from build123d import *

# Parameters (mm, degrees)
F1_DEPTH  = 22.5
F3_W      = 26.150945574
F3_H      = 2.773584798
F4_DEPTH  = 18
F7_R      = 5
F6_W      = 35.4622639716
F6_H      = 18.6226405203
F8_DEPTH  = 1.5
F10_R     = 2.7697383404
F11_DEPTH = 1.5
F14_R     = 2.5
F15_DEPTH = 1.3
F17_R     = 2.6497529256
F18_DEPTH = 1.5


# Not quite as in the source:
# - a pattern or mirror of a feature is missing from the dataset's text; its kind, count and spacing are read off the source's solid


with BuildPart() as f1:
    # F0 (on Front) → F1 (new body, symmetric)
    with BuildSketch(Plane.XZ):
        Polygon((9.8066031933, -27.5377351791), (14.9575471878, -27.5377351791), (14.9575471878, 27.5377351791), (-14.9575471878, 27.5377351791), (-14.9575471878, -27.5377351791), (2.2783020977, -27.5377351791), (2.2783020977, -14.8584917188), (9.8066031933, -14.8584917188), align=None)
    extrude(amount=F1_DEPTH, both=True)

    # F3 (on offset) → F4 (cut)
    with BuildSketch(Plane.XY.offset(27.5377351791)):
        with Locations((0, 15.5518874526)):
            Rectangle(F3_W, F3_H)
        with Locations((0, 5.5518874526)):
            Rectangle(F3_W, F3_H)
        with Locations((0, -4.4481125474)):
            Rectangle(F3_W, F3_H)
        with Locations((0, -14.4481125474)):
            Rectangle(F3_W, F3_H)
    extrude(amount=-F4_DEPTH, mode=Mode.SUBTRACT)

    # F7
    f7_edges = [f1.edges().sort_by_distance(p)[0] for p in [
        (0, -22.5, 27.537735),
        (0, 22.5, 27.537735),
    ]]
    fillet(f7_edges, radius=F7_R)

    # F6 (on offset) → F8 (cut)
    with BuildSketch(Plane(origin=(-14.9575471878, 0, 0), x_dir=(0, -1, 0), z_dir=(-1, 0, 0))):
        with Locations((0, 14.6603807807)):
            Rectangle(F6_W, F6_H)
    extrude(amount=-F8_DEPTH, mode=Mode.SUBTRACT)

    # F10 (on offset) → F11 (join)
    with BuildSketch(Plane(origin=(-13.4575471878, 0, 0), x_dir=(0, -1, 0), z_dir=(-1, 0, 0))):
        with Locations((-8.6189499125, 18.3801390231)):
            Circle(F10_R)
        with Locations((8.6189499125, 18.3801390231)):
            Circle(F10_R)
        with BuildLine():
            Line((3.3579913629, 12.3015097342), (-3.90234219, 12.3015097342))
            ThreePointArc((-3.90234219, 12.3015097342), (-0.2721754136, 8.6713429578), (3.3579913629, 12.3015097342))
        make_face()
    extrude(amount=F11_DEPTH)

    # F13 (on offset) + F14 (on offset) → F15 (join)
    with BuildSketch(Plane(origin=(-14.9575471878, 0, 0), x_dir=(0, -1, 0), z_dir=(-1, 0, 0))):
        Polygon((-12.6108881086, -15.9375003353), (-7.5907266326, -15.9375003353), (-7.5907266326, -10.8266131394), (-2.5705651566, -10.8266131394), (-2.5705651566, -5.7157259434), (-7.5907266326, -5.7157259434), (-7.5907266326, -0.9375003353), (-12.6108881086, -0.9375003353), (-12.6108881086, -5.7157259434), (-17.5705651566, -5.7157259434), (-17.5705651566, -10.8266131394), (-12.6108881086, -10.8266131394), align=None)
    with BuildSketch(Plane(origin=(-14.9575471878, 0, 0), x_dir=(0, -1, 0), z_dir=(-1, 0, 0))):
        with Locations((10.3680184111, -5.60903208)):
            Circle(F14_R)
        with Locations((4.8680184111, -15.1353115216)):
            Circle(F14_R)
        with Locations((15.8680184111, -15.1353115216)):
            Circle(F14_R)
    extrude(amount=F15_DEPTH)

    # F17 (on offset) → F18 (cut)
    with BuildSketch(Plane(origin=(0, 22.5, 0), x_dir=(-1, 0, 0), z_dir=(0, 1, 0))):
        with Locations((0, 18.2300075523)):
            Circle(F17_R)
        with Locations((8.105232894, 12.3412111554)):
            Circle(F17_R)
        with Locations((5.0093094152, 2.8129384324)):
            Circle(F17_R)
        with Locations((-5.0093094152, 2.8129384324)):
            Circle(F17_R)
        with Locations((-8.105232894, 12.3412111554)):
            Circle(F17_R)
    f18 = extrude(amount=-F18_DEPTH, mode=Mode.SUBTRACT)

    # F18_copies: F18 across plane
    add(f18.mirror(Plane(origin=(0, 0, 0), x_dir=(0, 0, -1), z_dir=(0, -1, 0))), mode=Mode.SUBTRACT)


solid = f1.part
Design review of the part built by this model. Coordinates are the model's own, in mm. A direction names the side the tool comes from. Give positions to 0.01 mm unless a question says otherwise; leave off trailing zeros. Order: outer loops, then holes, each group sorted by start corner. A loop starts at its lowest first (then second) coordinate and runs counter-clockwise, first axis right, second up. Notation, with made-up numbers: (-0.5, -24.5) - (36.5, -24.5) arc R28 ccw to (36.5, -1.5) - close; hole circle Ø4 at (59.25, 73.5). An arc over 180 degrees is marked (long way). Use CSV: the item, a comma, the result in double quotes. Start each with the question number.
Q1. For line 1 (Y direction, x = 10.5, z = 22.5); line 2 (Y direction, x = -1.5, z = 16.5); line 3 (X direction, y = 5.5, z = -24), list the stretches that pass through material, from the lowest coordinate up.
Q2. Take a section at C-C (y = 20). State the section outline as (x, z) points, and give its area (3 significant figures).
Q3. Take a section at D-D (z = 11.5). Count the separate pieces of the cut face and the enclosed holes in it, and give its area (3 significant figures).
Q4. Draft analysis for pull direction Z (two halves, no side actions). For faces 1 (the face through (-14.958, 0, 11)), 2 (the face through (-14.197, 10.817, 16.695)), 3 (the face through (-15.6, -10.04, -3.13)), state which applies: pulls with the +Z half, pulls with the -Z half, needs draft (parallel to the pull), parting line crosses it, or undercut.
Q5. Take a section at A-A (z = -21.5). State the section outline as (x, y) points, and give its area (3 significant figures).
Q6. Machinability: for faces 4 (the face through (-16, 5, -5.716)), 5 (the face through (0, -5.835, 19)), 6 (the face through (6.88, 21.76, 9.99)), 7 (the face through (5, -21, 3)), which of the approach directions +Z, -Z, +X, -X, +Y, -Y give a long, thin tool a straight path to every point of the face, cutting with its end or side? Answer none if there is none.
Q7. For P1, Ø3, axis at x = -8.11, z = 12.34, coming from the -Y side; P2, Ø1.4, axis at y = 15.5, z = 15.5, coming from the -X side; P3, Ø1, axis at y = 17.5, z = -20.5, coming from the -X side, all flat-tipped, find the tip position at first contact; note any pin that passes through.
Calculated:
1,line 1,"y = -22.5 to -15.83, -13.06 to -5.83, -3.06 to 4.17, 6.94 to 14.17, 16.94 to 22.5"
1,line 2,"y = -21 to -15.83, -13.06 to -5.83, -3.06 to 4.17, 6.94 to 14.17, 16.94 to 21"
1,line 3,"x = -14.96 to 2.28, 9.81 to 14.96"
2,outline,"(-14.96, -27.54) - (2.28, -27.54) - (2.28, -14.86) - (9.81, -14.86) - (9.81, -27.54) - (14.96, -27.54) - (14.96, 26.87) - (-14.96, 26.87) - close"
2,area,"1,530 mm²"
3,separate pieces,"1"
3,enclosed holes,"4"
3,area,"983 mm²"
4,face 1,"needs draft"
4,face 2,"undercut"
4,face 3,"parting line crosses it"
5,outline,"(-14.96, -22.5) - (2.28, -22.5) - (2.28, 22.5) - (-14.96, 22.5) - close; (9.81, -22.5) - (14.96, -22.5) - (14.96, 22.5) - (9.81, 22.5) - close"
5,area,"1,010 mm²"
6,face 4,"+Z, -X"
6,face 5,"+Z"
6,face 6,"+Y"
6,face 7,"-Y"
7,P1,"stops at y = -21"
7,P2,"stops at x = -13.46"
7,P3,"stops at x = -14.96"
